Geometry check sheet. Reference: the model listing, model coordinates, mm. Round coordinates to 2 decimals unless told otherwise and drop trailing zeros. Write item = value, one per line.
```python
from build123d import *

# Parameters (mm, degrees)
SKETCH_1_R          = 1.65
EXTRUDE_1_DEPTH     = 3
CUT_EXTRUDE_1_DEPTH = 3
FILLET_1_R          = 10
EXTRUDE_2_DEPTH     = 3
FILLET_2_R          = 10
SKETCH_6_R          = 1.65
CUT_EXTRUDE_2_DEPTH = 33
FILLET_3_R          = 10
FILLET_4_R          = 10
EXTRUDE_3_DEPTH     = 3
SKETCH_8_R          = 1.65
CUT_EXTRUDE_3_DEPTH = 4
CUT_EXTRUDE_5_DEPTH = 4
FILLET_6_R          = 15
FILLET_7_R          = 15
CUT_EXTRUDE_6_DEPTH = 4
FILLET_8_R          = 3
CUT_EXTRUDE_7_DEPTH = 4
FILLET_11_R         = 2
FILLET_12_R         = 10
CUT_EXTRUDE_8_DEPTH = 4
FILLET_13_R         = 10


with BuildPart() as part:
    # 草图1 → 凸台-拉伸1 (new body)
    with BuildSketch(Plane.XY):
        with BuildLine():
            Line((0, -30), (-76.636599455, -43.513100194))
            Line((-76.636599455, -43.513100194), (-94.295597777, -47.000187555))
            Line((-94.295597777, -47.000187555), (6.073993177, -158.471911377))
            Line((6.073993177, -158.471911377), (28.368337941, -138.397993186))
            Line((28.368337941, -138.397993186), (-11.934165547, -93.637528433))
            ThreePointArc((-11.934165547, -93.637528433), (-15.981640549, -73.743553217), (-0.54423259, -60.558761246))
            Line((-0.54423259, -60.558761246), (29, -55.349315916))
            Line((29, -55.349315916), (29, -50))
            Line((29, -50), (29, 0))
            Line((29, 0), (0, 0))
            Line((0, 0), (0, -30))
        make_face()
        with Locations((14.5, -15)):
            Circle(SKETCH_1_R, mode=Mode.SUBTRACT)
        with Locations((14.5, -45)):
            Circle(SKETCH_1_R, mode=Mode.SUBTRACT)
    extrude(amount=EXTRUDE_1_DEPTH)

    # 草图2 → 切除-拉伸1 (cut)
    with BuildSketch(Plane.XY.offset(3)):
        Polygon((-37.509702142, -36.613972526), (-44.1108023, -102.736049466), (-92.232515274, -102.736049466), (-120.974922517, -15.648301308), align=None)
    extrude(amount=-CUT_EXTRUDE_1_DEPTH, mode=Mode.SUBTRACT)

    # 圆角1
    fillet_1_edges = [part.edges().sort_by_distance(p)[0] for p in [
        (0, 0, 1.5),
        (29, 0, 1.5),
        (29, -55.349315916, 1.5),
        (28.368337941, -138.397993186, 1.5),
        (6.073993177, -158.471911377, 1.5),
        (0, -30, 1.5),
        (-37.509702142, -36.613972526, 1.5),
        (-44.1108023, -102.736049466, 1.5),
    ]]
    fillet(fillet_1_edges, radius=FILLET_1_R)

    # 草图3 → 凸台-拉伸2 (add)
    with BuildSketch(Plane.XY.offset(3)):
        Polygon((-15.981640549, -73.743553217), (19.461958696, -128.506456934), (-25.512326967, -91.299735006), align=None)
    extrude(amount=-EXTRUDE_2_DEPTH)

    # 圆角2
    fillet_2_edges = [part.edges().sort_by_distance(p)[0] for p in [
        (-15.981640549, -73.743553217, 1.5),
        (19.461958696, -128.506456934, 1.5),
    ]]
    fillet(fillet_2_edges, radius=FILLET_2_R)

    # 草图6 → 切除-拉伸2 (cut)
    with BuildSketch(Plane.XY):
        Polygon((-87.672076615, -95.352784266), (10.45531874, -167.066930238), (-55.522232913, -72.841221354), align=None)
        Polygon((-17.568683959, -74.741102773), (35.029880069, -149.859637147), (-14.273329758, -72.43367092), align=None)
        with Locations((-31.747162049, -80.643839485)):
            Circle(SKETCH_6_R)
        with Locations((-14.539868958, -105.218400814)):
            Circle(SKETCH_6_R)
        with Locations(Location((2.667424132, -129.792962143, 0), (0, 0, 180))):
            Circle(SKETCH_6_R)
    extrude(amount=CUT_EXTRUDE_2_DEPTH, mode=Mode.SUBTRACT)

    # 圆角3
    # the kernel refuses this fillet: 10 mm, written as the material it adds along each edge
    with BuildSketch(Plane(origin=(-17.568683959, -74.741102773, 0), x_dir=(0.8191520442890025, 0.5735764363510307, 0), z_dir=(0, 0, 1))) as fillet_3_piece_1:
        with BuildLine():
            CenterArc((10, -8.017112469), FILLET_3_R, 126.706173487, 53.293826513)
            Line((0, -8.017112469), (-0.2, -8.017112469))
            Line((-0.2, -8.017112469), (-0.2, 0))
            Line((-0.2, 0), (0, 0.2))
            ThreePointArc((0, 0.2), (2.011442335, 0.2), (3.903342364, 0.160342249))
            Line((3.903342364, 0.160342249), (4.02288467, 0))
        make_face()
    extrude(amount=3)

    # 圆角4
    fillet_4_edges = [part.edges().sort_by_distance(p)[0] for p in [
        (-42.922716134, -90.835196128, 1.5),
    ]]
    fillet(fillet_4_edges, radius=FILLET_4_R)

    # 草图7 → 凸台-拉伸3 (add)
    with BuildSketch(Plane.XY.offset(3)):
        Polygon((-34.566125117, -102.769644932), (-65.373370144, -58.772339354), (-42.090796033, -16.519494834), (-31.58573936, -35.55781759), align=None)
    extrude(amount=-EXTRUDE_3_DEPTH)

    # 草图8 → 切除-拉伸3 (cut)
    with BuildSketch(Plane.XY.offset(3)):
        with Locations((-48.954455139, -56.069278157)):
            Circle(SKETCH_8_R)
    extrude(amount=-CUT_EXTRUDE_3_DEPTH, mode=Mode.SUBTRACT)

    # 草图9 → 切除-拉伸5 (cut)
    with BuildSketch(Plane.XY.offset(3)):
        Polygon((-31.58573936, -35.55781759), (-42.090796033, -16.519494834), (-65.373370144, -58.772339354), align=None)
    extrude(amount=-CUT_EXTRUDE_5_DEPTH, mode=Mode.SUBTRACT)

    # 圆角6
    fillet_6_edges = [part.edges().sort_by_distance(p)[0] for p in [
        (-65.373370144, -58.772339354, 1.5),
    ]]
    fillet(fillet_6_edges, radius=FILLET_6_R)

    # 圆角7
    # the kernel refuses this fillet: 15 mm, written as the material it takes off along each edge
    with BuildSketch(Plane(origin=(-31.58573936, -35.55781759, 7.815831315), x_dir=(-0.8242067246408917, -0.5662890384394996, 0), z_dir=(0, 0, -1))) as fillet_7_piece_1:
        with BuildLine():
            CenterArc((1.926332526, -15), FILLET_7_R, 90, 7.049103332)
            Line((0.085533646, -0.11337985), (0, 0))
            Line((0, 0), (1.926332526, 0))
        make_face()
    extrude(amount=12.63166263, mode=Mode.SUBTRACT)

    # 草图10 → 切除-拉伸6 (cut)
    with BuildSketch(Plane.XY.offset(3)):
        Polygon((-31.497161439, -67.881768792), (-15.547904948, -44.140451067), (-33.616807091, -45.881308748), align=None)
        Polygon((-13.635910341, -59.04618523), (3.278405873, -49.224969364), (-4.542191946, -39.403753498), align=None)
        Polygon((10.242872605, -36.716551154), (23.145942056, -29.046782931), (10.242872605, -21.377014708), align=None)
        Polygon((-47.382252639, -78.462252302), (-36.982602957, -68.475134443), (-43.961583104, -62.806110969), align=None)
        Polygon((-31.497161439, -98.196884234), (-13.635910341, -92.671187293), (-21.595666913, -84.382641882), align=None)
        Polygon((-14.194825195, -122.494735697), (1.82276298, -116.352745612), (-5.544832941, -108.458892839), align=None)
        Polygon((4.547829517, -147.416387444), (16.294826397, -140.502022472), (10.242872605, -133.5876575), align=None)
    extrude(amount=-CUT_EXTRUDE_6_DEPTH, mode=Mode.SUBTRACT)

    # 圆角8
    fillet_8_edges = [part.edges().sort_by_distance(p)[0] for p in [
        (16.294826397, -140.502022472, 1.5),
        (4.547829517, -147.416387444, 1.5),
        (10.242872605, -133.5876575, 1.5),
        (1.82276298, -116.352745612, 1.5),
        (-14.194825195, -122.494735697, 1.5),
        (-5.544832941, -108.458892839, 1.5),
        (-13.635910341, -92.671187293, 1.5),
        (-31.497161439, -98.196884234, 1.5),
        (-21.595666913, -84.382641882, 1.5),
        (-36.982602957, -68.475134443, 1.5),
        (-47.382252639, -78.462252302, 1.5),
        (-43.961583104, -62.806110969, 1.5),
        (23.145942056, -29.046782931, 1.5),
        (10.242872605, -36.716551154, 1.5),
        (10.242872605, -21.377014708, 1.5),
        (3.278405873, -49.224969364, 1.5),
        (-13.635910341, -59.04618523, 1.5),
        (-4.542191946, -39.403753498, 1.5),
        (-15.547904948, -44.140451067, 1.5),
        (-31.497161439, -67.881768792, 1.5),
        (-33.616807091, -45.881308748, 1.5),
    ]]
    fillet(fillet_8_edges, radius=FILLET_8_R)

    # 草图13 → 切除-拉伸7 (cut)
    with BuildSketch(Plane.XY.offset(3)):
        with BuildLine():
            ThreePointArc((2.619259417, -15), (4.083725511, -11.464466094), (7.619259417, -10))
            Line((7.619259417, -10), (22.619259417, -10))
            ThreePointArc((22.619259417, -10), (26.154793323, -11.464466094), (27.619259417, -15))
            Line((27.619259417, -15), (27.619259417, -49.552905051))
            ThreePointArc((27.619259417, -49.552905051), (26.154793323, -53.088438957), (22.619259417, -54.552905051))
            Line((22.619259417, -54.552905051), (2.619259417, -54.552905051))
            Line((2.619259417, -54.552905051), (2.619259417, -60.000952252))
            Line((2.619259417, -60.000952252), (20.736481777, -56.806397134))
            ThreePointArc((20.736481777, -56.806397134), (26.660444431, -53.386195701), (29, -46.958319604))
            Line((29, -46.958319604), (29, -10))
            ThreePointArc((29, -10), (26.071067812, -2.928932188), (19, 0))
            Line((19, 0), (10, 0))
            ThreePointArc((10, 0), (2.928932188, -2.928932188), (0, -10))
            Line((0, -10), (0, -15))
            Line((0, -15), (2.619259417, -15))
        make_face()
    extrude(amount=-CUT_EXTRUDE_7_DEPTH, mode=Mode.SUBTRACT)

    # 圆角11
    fillet_11_edges = [part.edges().sort_by_distance(p)[0] for p in [
        (2.619259417, -60.000952252, 1.5),
        (2.619259417, -54.552905051, 1.5),
    ]]
    fillet(fillet_11_edges, radius=FILLET_11_R)

    # 圆角12
    # the kernel refuses this fillet: 10 mm, written as the material it takes off along each edge
    with BuildSketch(Plane(origin=(0, -15, 19.695908746), x_dir=(1, 0, 0), z_dir=(0, 0, -1))) as fillet_12_piece_1:
        with BuildLine():
            CenterArc((9.999518916, 6.7477233), FILLET_12_R, 180.397405601, 42.039067217)
            Line((-0.000240542, 6.678363494), (-1.000216488, 6.671427514))
            ThreePointArc((-1.000216488, 6.671427514), (-1, 6.609003688), (-1, 0))
            Line((-1, 0), (0, -1))
            ThreePointArc((0, -1), (1.309629709, -1), (1.881233468, -0.67477233))
            Line((1.881233468, -0.67477233), (2.619259417, 0))
        make_face()
    extrude(amount=36.391817492, mode=Mode.SUBTRACT)

    # 草图14 → 切除-拉伸8 (cut)
    with BuildSketch(Plane.XY.offset(3)):
        Polygon((2.619259417, -15), (2.619259417, -31.018717886), (-8.263518223, -31.457081218), (-8.263518223, -7.080960467), align=None)
    extrude(amount=-CUT_EXTRUDE_8_DEPTH, mode=Mode.SUBTRACT)

    # 圆角13
    fillet_13_edges = [part.edges().sort_by_distance(p)[0] for p in [
        (2.619259417, -31.018717886, 1.5),
    ]]
    fillet(fillet_13_edges, radius=FILLET_13_R)


solid = part.part
```
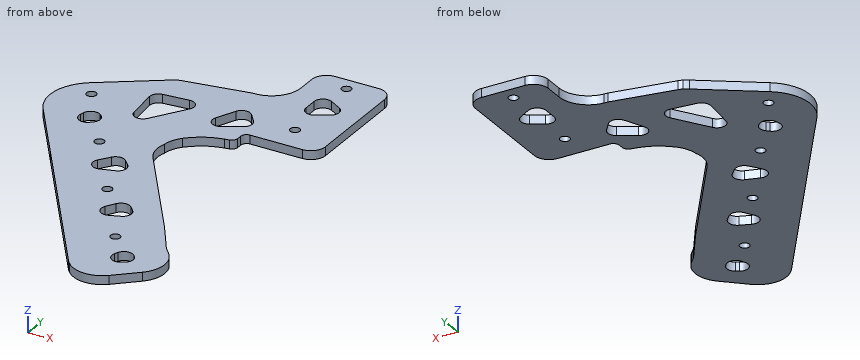
(1) Section check A-A (z = 1). State how many separate pieces and enclosed holes the cut face has, then the cut area to 3 significant figures.
Answers follow:
separate_pieces = 1
enclosed_holes = 13
area = 5,220 mm²
(2) Gauge pin test, flat ends, axial feed: pin 1 (1.5 mm diameter, centred on x = -17, z = 2.5, fed in from -Y); pin 2 (1.4 mm diameter, centred on y = -57, z = 1, fed in from +X); pin 3 (1.5 mm diameter, centred on x = 9.5, z = 1, fed in from -Y). Record the tip position at first contact, or that the pin passes through.
Answers follow:
pin_1 = -128.93
pin_2 = 2.64
pin_3 = -154.16
(3) Scan lines: L1, parallel to X at y = -112.5, z = 2.6; L2, parallel to X at y = -21, z = 1.55; L3, parallel to Y at x = -24, z = 0.8. Record each from-to range of solid material in increasing order. Write a range as [from, to].
Answers follow:
L1 = [-27.75, -8.04], [-1.77, 8.87]
L2 = [2.62, 27.62]
L3 = [-117.86, -95.69], [-87.74, -56.72], [-44.95, -34.23]
